Can you work these out from the model? Positions are in its coordinate system, mm. A direction names the side the tool comes from. Round coordinates to 2 decimals unless told otherwise and drop trailing zeros. Order: outer loops, then holes, each group sorted by start corner. A loop starts at its lowest first (then second) coordinate and runs counter-clockwise, first axis right, second up. Notation, with made-up numbers: M 11,48.5 L 34,48.5 A18 ccw 34,79.5 Z; hole C -36.75,13.5 d10. An arc over 180 degrees is marked long. One line per question, with ' | ' between items.
Autodesk Inventor part; units mm, degrees
ref_plane "YZ Plane" through (0, 0, 0) normal (1, 0, 0) x (0, 1, 0)
ref_plane "XZ Plane" through (0, 0, 0) normal (0, 1, 0) x (-1, 0, 0)
ref_plane "XY Plane" through (0, 0, 0) normal (0, 0, 1) x (1, 0, 0)
sketch "Sketch1" plane through (0, 0, 0) normal (0, 1, 0) x (-1, 0, 0)
  circle A0 centre (65, 195) radius 12
  circle A1 centre (65, -195) radius 12
  circle A2 centre (-65, 195) radius 12
  circle A3 centre (-65, -195) radius 12
  line L0 (77, 195) -> (77, -195)
  line L1 (65, -207) -> (-65, -207)
  line L2 (65, 207) -> (-65, 207)
  line L3 (-77, 195) -> (-77, -195)
  line L4 (73, 195) -> (73, -195)
  circle A4 centre (65, 195) radius 8
  line L5 (65, 203) -> (-65, 203)
  circle A5 centre (-65, 195) radius 8
  line L6 (-73, 195) -> (-73, -195)
  circle A6 centre (-65, -195) radius 8
  line L7 (65, -203) -> (-65, -203)
  circle A7 centre (65, -195) radius 8
  point P0 (0, 0)
  point P1 (77, 0)
  point P2 (0, 207)
  point P3 (35, 143)
  point P4 (68, 135)
  point P5 (68, -135)
  point P6 (35, -143)
  point P7 (-60, -203)
  point P8 (-68, -135)
  point P9 (-68, 135)
  point P10 (-60, 203)
  dimension "d0" = 24
  dimension "d1" = 24
  dimension "d2" = 24
  dimension "d3" = 24
  dimension "d6" = 4
  dimension "d7" = 4
  dimension "d8" = 4
  dimension "d9" = 4
  dimension "d10" = 4
  dimension "d11" = 4
  dimension "d12" = 4
  dimension "d13" = 4
  dimension "d35" = 414
  dimension "d36" = 154
extrude "Extrusion1" add sketch "Sketch1" along normal blind 4.5 contours A0 L4 A4 L5 | L0 A1 L4 A0 | A0 L5 A2 L2 | A1 L7 A7 L4 | A2 L5 A5 L6 | L1 A3 L7 A1 | A2 L6 A3 L3 | A3 L6 A6 L7 picked at (59.6594, 203.5636) picked at (59.6594, -203.5636) picked at (-59.6594, 203.5636) picked at (-59.6594, -203.5636)
sketch "Sketch2" plane through (0, 4.5, 0) normal (0, 1, 0) x (1, 0, 0)
  line L0 (-77, 195) -> (-77, -195)
  arc A0 (-77, -195) -> (-65, -207) centre (-65, -195) ccw
  line L1 (-65, -207) -> (65, -207)
  arc A1 (65, -207) -> (77, -195) centre (65, -195) ccw
  line L2 (77, -195) -> (77, 195)
  arc A2 (77, 195) -> (65, 207) centre (65, 195) ccw
  line L3 (65, 207) -> (-65, 207)
  arc A3 (-65, 207) -> (-77, 195) centre (-65, 195) ccw
  line L4 (-74.5, -195) -> (-74.5, 195)
  arc A4 (-65, 204.5) -> (-74.5, 195) centre (-65, 195) ccw
  line L5 (-65, 204.5) -> (65, 204.5)
  arc A5 (74.5, 195) -> (65, 204.5) centre (65, 195) ccw
  line L6 (74.5, 195) -> (74.5, -195)
  arc A6 (65, -204.5) -> (74.5, -195) centre (65, -195) ccw
  line L7 (65, -204.5) -> (-65, -204.5)
  arc A7 (-74.5, -195) -> (-65, -204.5) centre (-65, -195) ccw
  line L8 (-75.5, -195) -> (-75.5, 195)
  arc A8 (-65, 205.5) -> (-75.5, 195) centre (-65, 195) ccw
  line L9 (-65, 205.5) -> (65, 205.5)
  arc A9 (75.5, 195) -> (65, 205.5) centre (65, 195) ccw
  line L10 (75.5, 195) -> (75.5, -195)
  arc A10 (65, -205.5) -> (75.5, -195) centre (65, -195) ccw
  line L11 (65, -205.5) -> (-65, -205.5)
  arc A11 (-75.5, -195) -> (-65, -205.5) centre (-65, -195) ccw
  point P0 (0, 0)
  dimension "d16" = 2.5
  dimension "d17" = 1.5
extrude "Extrusion2" cut sketch "Sketch2" against normal blind 1 contours L8 A8 L9 A9 L10 A10 L11 A11
chamfer "Chamfer3" distance 0.5 distance2 1 8 edges at (0, 4.5, 205.5) (-72.4246, 4.5, 202.4246) (-75.5, 4.5, 0) (-72.4246, 4.5, -202.4246) (0, 4.5, -205.5) (72.4246, 4.5, -202.4246) (75.5, 4.5, 0) (72.4246, 4.5, 202.4246) measured on face at (76, 4.5, -65)
chamfer "Chamfer4" distance 0.5 distance2 1 8 edges at (0, 4.5, 204.5) (71.7175, 4.5, 201.7175) (74.5, 4.5, 0) (71.7175, 4.5, -201.7175) (0, 4.5, -204.5) (-71.7175, 4.5, -201.7175) (-74.5, 4.5, 0) (-71.7175, 4.5, 201.7175) measured on face at (-74, 4.5, -65)
chamfer "Chamfer5" distance 0.5 angle 45 32 edges at (0, 4.5, 207) (73.4853, 4.5, 203.4853) (77, 4.5, 0) (73.4853, 4.5, -203.4853) (0, 4.5, -207) (-73.4853, 4.5, -203.4853) (-77, 4.5, 0) (-73.4853, 4.5, 203.4853) (0, 4.5, 203) (-70.6569, 4.5, 200.6569) (-73, 4.5, 0) (-70.6569, 4.5, -200.6569) (0, 4.5, -203) (70.6569, 4.5, -200.6569) (73, 4.5, 0) (70.6569, 4.5, 200.6569) (73.4853, 0, 203.4853) (77, 0, 0) (73.4853, 0, -203.4853) (0, 0, -207) (-73.4853, 0, -203.4853) (-77, 0, 0) (-73.4853, 0, 203.4853) (0, 0, 207) (0, 0, 203) (-70.6569, 0, 200.6569) (-73, 0, 0) (-70.6569, 0, -200.6569) (0, 0, -203) (70.6569, 0, -200.6569) (73, 0, 0) (70.6569, 0, 200.6569)
properties part number "LI0005-SEAL"
(1) Please list where these lines run through material, in increasing order: probe 1 along Z at (x, y) = (-20, 3.3); probe 2 along X at (y, z) = (2.25, -189.5); probe 3 along X at (y, z) = (3.7, 132). Write a range as [from, to].
Final values:
probe 1: [-207, -203], [203, 207] | probe 2: [-77, -73], [73, 77] | probe 3: [-77, -75.6], [-74.4, -73], [73, 74.4], [75.6, 77]
(2) Thinking about a two-plate mould opening in Z: for faces 1 (the flat face through (74, 0, 1)), 2 (the conical face through (-73.32, 4.36, -203.14)), 3 (the conical face through (70.82, 0.36, 200.69)), which applies, released by +Z, released by -Z, zero draft, split by the parting line, or undercut?
Final values:
face 1: zero draft | face 2: released by -Z | face 3: undercut
(3) If we section it at B-B on y = 2.05: Please give me the cut outline in (x, z), plus the area to 3 significant figures.
Final values:
outline: M -77,-195 A12 ccw -65,-207 L 65,-207 A12 ccw 77,-195 L 77,195 A12 ccw 65,207 L -65,207 A12 ccw -77,195 Z; hole M -73,-195 A8 ccw -65,-203 L 65,-203 A8 ccw 73,-195 L 73,195 A8 ccw 65,203 L -65,203 A8 ccw -73,195 Z | area: 4,410 mm^2
(4) On a 3-axis mill with a long thin cutter (end or side, diameter ignored), from which of +Z, -Z, +X, -X, +Y, -Y can I reach the whole of each face in a straight line? I mean faces 4 (the conical face through (73.32, 4.36, 203.14)), 5 (the cylindrical face through (-70.719, 2.226, -200.594)), 6 (the conical face through (71.5, 4.33, 201.35)), 7 (the conical face through (73.32, 0.14, -203.14)), 8 (the conical face through (-70.69, 0.36, 200.82)). Say none if no direction works.
Final values:
face 4: +Z, +X, +Y | face 5: +Y, -Y | face 6: +Y | face 7: -Z, +X, -Y | face 8: -Y
